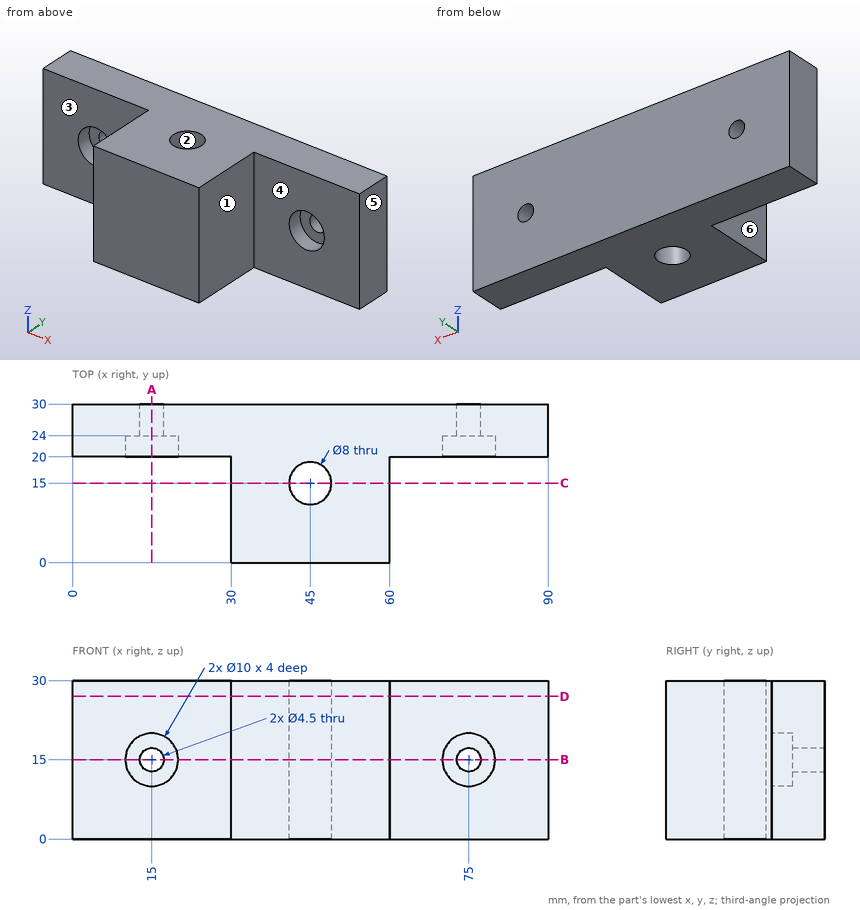
Here's the drawing with two shaded views (mm, measured from the low corner). I have some questions. A direction names the side the tool comes from. Coordinates: 2 decimals unless noted, no trailing zeros. Order: outer loops, then holes, each group sorted by start corner. A loop starts at its lowest first (then second) coordinate and runs counter-clockwise, first axis right, second up.
Item 1: If we section it at B-B on z = 15: List the corners of the cut face in (x, y) for me.
Result sheet:
outline: (0, 20) - (10, 20) - (10, 24) - (12.75, 24) - (12.75, 30) - (0, 30) - close; (17.25, 24) - (20, 24) - (20, 20) - (30, 20) - (30, 0) - (60, 0) - (60, 20) - (70, 20) - (70, 24) - (72.75, 24) - (72.75, 30) - (17.25, 30) - close; (77.25, 24) - (80, 24) - (80, 20) - (90, 20) - (90, 30) - (77.25, 30) - close; hole circle Ø8 at (45, 15)
Item 2: For the marked faces 4, 5 and 6, which set-ups out of +Z, -Z, +X, -X, +Y, -Y let a thin tool reach every point of the face, with its end or its side?
Result sheet:
face 4: +Z, -Z, +X, -Y
face 5: +Z, -Z, +X, +Y, -Y
face 6: +Z, -Z, -X, -Y
Item 3: If we section it at D-D on z = 27: List the corners of the cut face in (x, y) for me.
Result sheet:
outline: (0, 20) - (30, 20) - (30, 0) - (60, 0) - (60, 20) - (90, 20) - (90, 30) - (0, 30) - close; hole circle Ø8 at (45, 15)
Item 4: I need wall thicknesses on line 1 (X direction, y = 22, z = 15.25); line 2 (X direction, y = 26.65, z = 15); line 3 (Z direction, x = 75, y = 27). Which ranges of each line are inside material? Lowest first, please.
Result sheet:
line 1: x = 0 to 10.01, 19.99 to 70.01, 79.99 to 90
line 2: x = 0 to 12.75, 17.25 to 72.75, 77.25 to 90
line 3: z = 0 to 12.75, 17.25 to 30
Item 5: If we section it at C-C on y = 15: List the corners of the cut face in (x, z) for me, plus the area to 3 significant figures.
Result sheet:
outline: (30, 0) - (41, 0) - (41, 30) - (30, 30) - close; (49, 0) - (60, 0) - (60, 30) - (49, 30) - close
area: 660 mm2
Item 6: If we mould it in two halves opening along X, with no side actions, what happens to the marked faces 1, 2 and 3? For each: +X half, -X half, draft (parallel to the pull), parting line (faces both ways), or undercut.
Result sheet:
face 1: +X half
face 2: undercut
face 3: draft
Item 7: If we section it at A-A on x = 15: List the corners of the cut face in (y, z) for me.
Result sheet:
outline: (20, 0) - (30, 0) - (30, 12.75) - (24, 12.75) - (24, 10) - (20, 10) - close; (20, 20) - (24, 20) - (24, 17.25) - (30, 17.25) - (30, 30) - (20, 30) - close
Item 8: For P1, Ø8, axis at x = 15, z = 15, coming from the -Y side; P2, Ø9, axis at x = 81, z = 8.5, coming from the -Y side; P3, Ø10, axis at y = 11, z = 18.5, coming from the +X side, each with a flat end and sliding along its axis, tell me the tip position at first contact or that it passes through.
Result sheet:
P1: stops at y = 24
P2: stops at y = 20
P3: stops at x = 60
